Source: CAD feature listing. Evaluate the final solid. Frame: model axes, mm. Face numbers are marked on the shaded views. A direction names the side the tool comes from. Give positions to 0.01 mm unless a question says otherwise; leave off trailing zeros. Order: outer loops, then holes, each group sorted by start corner. A loop starts at its lowest first (then second) coordinate and runs counter-clockwise, first axis right, second up.
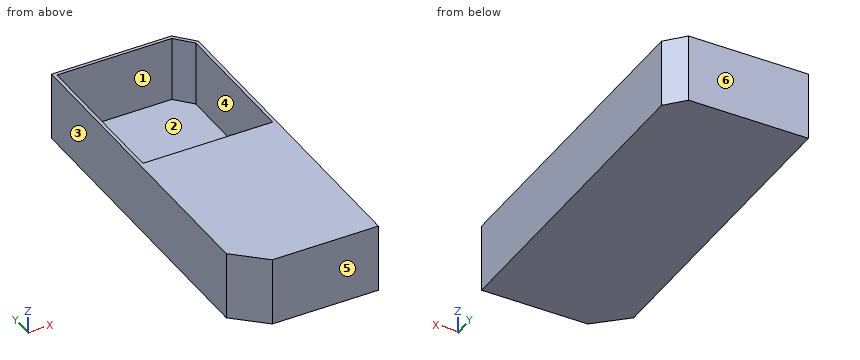
from build123d import *

# Parameters (mm, degrees)
F1_DEPTH = 31.75
F3_DEPTH = 60.325
F5_DEPTH = 3.175


with BuildPart() as f1:
    # F0 (on Top) → F1 (new body, symmetric)
    with BuildSketch(Plane.XY):
        Polygon((63.5, 141.6507737828), (47.9251928627, 158.75), (-63.5, 158.75), (-63.5, -132.9134553671), (-35.1417474449, -158.75), (63.5, -158.75), align=None)
    extrude(amount=F1_DEPTH, both=True)

    # F2 (on face) → F3 (cut)
    with BuildSketch(Plane.XY.offset(31.75)):
        Polygon((-60.325, -131.5109922598), (-33.9122881347, -155.575), (60.325, -155.575), (60.325, 140.4215420307), (46.5224932469, 155.575), (-60.325, 155.575), align=None)
    extrude(amount=-F3_DEPTH, mode=Mode.SUBTRACT)

    # F4 (on face) → F5 (join)
    with BuildSketch(Plane.XY.offset(31.75)):
        Polygon((60.325, 12.0320038701), (-60.325, 12.0320038701), (-60.325, -131.5109922598), (-33.9122881347, -155.575), (60.325, -155.575), align=None)
    extrude(amount=-F5_DEPTH)


solid = f1.part
1) Reachability of the marked faces 1, 2 and 3 from +Z, -Z, +X, -X, +Y, -Y: full face, straight path, thin tool, end or side. Return the list, or none.
Checks:
face 1: +Z
face 2: none
face 3: +Z, -Z, -X, +Y, -Y
2) Section query D-D on x = 21.5. Output: boundary loops of the cut face in (y, z) (3 decimals).
Checks:
outline: (-158.75, -31.75) - (158.75, -31.75) - (158.75, 31.75) - (155.575, 31.75) - (155.575, -28.575) - (-155.575, -28.575) - (-155.575, 28.575) - (12.032, 28.575) - (12.032, 31.75) - (-158.75, 31.75) - close
3) Section query C-C on y = 106.5. Output: boundary loops of the cut face in (x, z) (3 decimals), and give its area (3 significant figures).
Checks:
outline: (-63.5, -31.75) - (63.5, -31.75) - (63.5, 31.75) - (60.325, 31.75) - (60.325, -28.575) - (-60.325, -28.575) - (-60.325, 31.75) - (-63.5, 31.75) - close
area: 786 mm2
4) Section query A-A on y = -76.5. Output: boundary loops of the cut face in (x, z) (3 decimals).
Checks:
outline: (-63.5, -31.75) - (63.5, -31.75) - (63.5, 31.75) - (-63.5, 31.75) - close; hole (-60.325, -28.575) - (60.325, -28.575) - (60.325, 28.575) - (-60.325, 28.575) - close
5) Pull-direction query (Y, two-part tool) for the marked faces 4, 5 and 6; classes: +Y half, -Y half, draft (parallel to the pull), parting line (faces both ways), or undercut.
Checks:
face 4: undercut
face 5: -Y half
face 6: +Y half
6) First-contact query: pin 1 Ø1.5 at (x, y) = (27, 50) entering from +Z (3 decimals). Flat tip, straight axial feed; report the tip coordinate or a pass-through.
Checks:
pin 1: stops at z = -28.575
7) Ray query, L1, parallel to Z at x = 8, y = -75.5 (3 decimals); L2, parallel to Y at x = -28, z = 13.5 (3 decimals); L3, parallel to X at y = 1, z = -7 (3 decimals). Return the intervals inside material, ascending.
Checks:
L1: z = -31.75 to -28.575, 28.575 to 31.75
L2: y = -158.75 to -155.575, 155.575 to 158.75
L3: x = -63.5 to -60.325, 60.325 to 63.5
